Could you check a few things on this model? Use its own coordinates, in mm. A direction names the side the tool comes from. Give positions to 0.01 mm unless a question says otherwise; leave off trailing zeros. Order: outer loops, then holes, each group sorted by start corner. A loop starts at its lowest first (then second) coordinate and runs counter-clockwise, first axis right, second up. Notation, with made-up numbers: M 23,63.5 L 78,63.5 A32 cw 78,92.5 Z; hole C -13.75,51.5 d10. An arc over 180 degrees is marked long. Use a Markdown table: item, result. Add a question column.
Item 1: If we mould it in two halves opening along Y, with no side actions, what happens to faces 1 (the face through (0, -11, -304.8)), 2 (the face through (-15.875, 0, 8)), 3 (the face through (0, -12.7, 8))? For each: released by +Y, released by -Y, zero draft, split by the parting line, or undercut.
Item 2: If I drill on L1, parallel to Y at x = -17, z = -266; L2, parallel to Y at x = -1, z = -70.5 (3 decimals); L3, parallel to X at y = -0.5, z = 173 (3 decimals), over which ranges is the centre line in solid material (lowest first)? Write a range as from..to.
Item 3: I'm going to push a flat-ended pin straight in: pin 1 Ø4 at (y, z) = (0, -266.7) entering from -X (3 decimals). Where does the tip first touch, or does it pass through?
Item 4: Suppose I cut it at B-B on z = -189. Write out the boundary of the cut face in (x, y) (3 decimals).
Item 5: Suppose I cut it at A-A on x = -7.5. Write out the boundary of the cut face in (y, z) (3 decimals), plus the area to 3 significant figures.
Item 6: For faces 4 (the face through (-19.05, 0, 8)), 5 (the face through (0, 9.525, 8)), which set-ups out of +Z, -Z, +X, -X, +Y, -Y let a thin tool reach every point of the face, with its end or its side?
from build123d import *

# Parameters (mm, degrees)
BOSS_EXTRUDE1_DEPTH      = 330.200001
BOSS_EXTRUDE1_DEPTH_BACK = 330.200001
SKETCH3_W                = 38.1
SKETCH3_H                = 25.4
SKETCH3_W_2              = 31.75
SKETCH3_H_2              = 19.05
F_10_CLEARANCE_HOLE1_D   = 4.9784


with BuildPart() as part:
    # Sketch3 → Boss-Extrude1 (new, two sides: drawn at the far end of the back side and taken through both)
    with BuildSketch(Plane.XY.offset(-BOSS_EXTRUDE1_DEPTH_BACK)):
        Rectangle(SKETCH3_W, SKETCH3_H)
        Rectangle(SKETCH3_W_2, SKETCH3_H_2, mode=Mode.SUBTRACT)
    extrude(amount=BOSS_EXTRUDE1_DEPTH + BOSS_EXTRUDE1_DEPTH_BACK)

    # SurfaceCut1
    split(bisect_by=Plane(origin=(0, 0, -304.800000508), x_dir=(-1, 0, 0), z_dir=(0, 0, -1)), keep=Keep.BOTTOM)

    # #10 Clearance Hole1 (through all)
    with Locations(Plane(origin=(19.05, 0, 0), x_dir=(0, 0, -1), z_dir=(1, 0, 0))):
        with Locations((-128.5875, 0), (-103.1875, 0), (77.787500575, 1.014e-06), (103.187500575, 1.014e-06), (-317.500000508, 0), (-292.100000508, 0), (266.700000508, 0), (292.100000508, 0)):
            Hole(F_10_CLEARANCE_HOLE1_D / 2)


solid = part.part
Findings below:
| question | item | result |
|---|---|---|
| 1 | face 1 | zero draft |
| 1 | face 2 | undercut |
| 1 | face 3 | released by -Y |
| 2 | L1 | y = -12.7..-2.39, 2.39..12.7 |
| 2 | L2 | y = -12.7..-9.525, 9.525..12.7 |
| 2 | L3 | x = -19.05..-15.875, 15.875..19.05 |
| 3 | pin 1 | passes through |
| 4 | outline | M -19.05,-12.7 L 19.05,-12.7 L 19.05,12.7 L -19.05,12.7 Z; hole M -15.875,-9.525 L 15.875,-9.525 L 15.875,9.525 L -15.875,9.525 Z |
| 5 | outline | M -12.7,-304.8 L -9.525,-304.8 L -9.525,330.2 L -12.7,330.2 Z; M 9.525,-304.8 L 12.7,-304.8 L 12.7,330.2 L 9.525,330.2 Z |
| 5 | area | 4,030 mm^2 |
| 6 | face 4 | +Z, -Z, -X, +Y, -Y |
| 6 | face 5 | +Z, -Z |
